Geometry: final body of the model. Coordinates: model frame, mm. Face numbers are marked on the shaded views. A direction names the side the tool comes from. Round coordinates to 2 decimals unless told otherwise and drop trailing zeros. Write each loop counter-clockwise with the first axis right and the second up, starting at its lowest first coordinate (ties: lowest second). Pieces come first, ordered by that corner, then holes. Notation, with made-up numbers: (78.5, -0.5) - (88.5, -0.5) arc R22 ccw to (88.5, 27.5) - close; hole circle Ø3 at (10, 12.25). An arc over 180 degrees is marked (long way). Use a Markdown table: item, result. Add a question column.
```python
from build123d import *

# Parameters (mm, degrees)
F0_R     = 28.575
F0_R_2   = 17.4625
F1_DEPTH = 61.976
F3_R     = 21.844
F4_DEPTH = 50.8
F7_R     = 1.5875
F8_DEPTH = 12.7


with BuildPart() as f1:
    # F0 (on Right) → F1 (new body)
    with BuildSketch(Plane.YZ):
        Circle(F0_R)
        Circle(F0_R_2, mode=Mode.SUBTRACT)
    extrude(amount=-F1_DEPTH)

    # F3 (on offset) → F4 (cut)
    with BuildSketch(Plane.YZ.offset(-5.588)):
        Circle(F3_R)
    extrude(amount=-F4_DEPTH, mode=Mode.SUBTRACT)

    # F7 (on face) → F8 (cut)
    with BuildSketch(Plane.XY.offset(28.575)):
        with Locations((-13.462, 0)):
            Circle(F7_R)
    extrude(amount=-F8_DEPTH, mode=Mode.SUBTRACT)


solid = f1.part
```
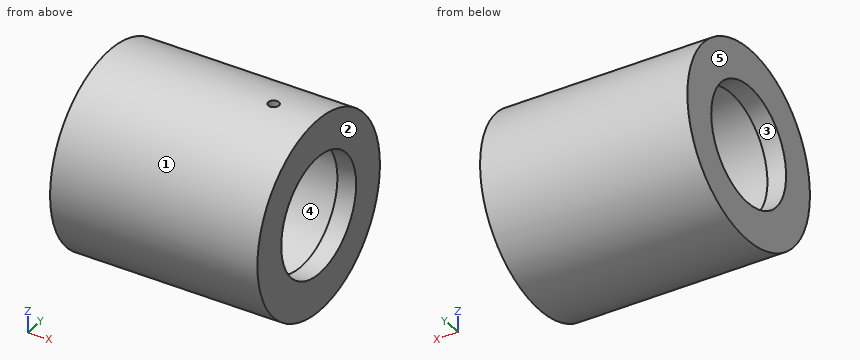
1) Section C-C, the plane y = -12. Return the cut outline in (x, z), then the cut area to 3 significant figures.
2) Set-up query: the marked faces 4 and 5. Return all of +Z, -Z, +X, -X, +Y, -Y with unobstructed straight access to the full face (end or side cutting, diameter ignored); none if empty.
3) Section B-B, the plane y = 0. Return the cut outline in (x, z) (1 decimal).
4) Material intervals for L1, parallel to X at y = 19.5, z = 8; L2, parallel to Z at x = -3.05, y = 0 (1 decimal); L3, parallel to Y at x = -11.5, z = -11.5, sorted ascending. Write a range as from..to.
5) Draft query along Z for the marked faces 1, 2 and 3. Return one class per face: released by +Z, released by -Z, zero draft, split by the parting line, or undercut.
6) Section A-A, the plane z = 0. Return the cut outline in (x, y) (1 decimal), then the cut area to 3 significant figures.
7) Pin query (flat end, axial travel): P1, Ø10, axis at x = -14, y = 6.5, coming from the +Z side; P2, Ø4, axis at x = -25, y = 7, coming from the -Z side; P3, Ø1.9, axis at x = -13.462, y = 0, coming from the +Z side; P4, Ø22, axis at y = 5.5, z = -1, coming from the -X side. Return the tip coordinate at first contact, or that it passes through.
8) Section D-D, the plane z = 23. Return the cut outline in (x, y) (1 decimal), then the cut area to 3 significant figures.
Output values:
| question | item | result |
|---|---|---|
| 1 | outline | (-61.98, -25.93) - (0, -25.93) - (0, -12.69) - (-5.59, -12.69) - (-5.59, -18.25) - (-56.39, -18.25) - (-56.39, -12.69) - (-61.98, -12.69) - close; (-61.98, 12.69) - (-56.39, 12.69) - (-56.39, 18.25) - (-5.59, 18.25) - (-5.59, 12.69) - (0, 12.69) - (0, 25.93) - (-61.98, 25.93) - close |
| 1 | area | 1,080 mm^2 |
| 2 | face 4 | none |
| 2 | face 5 | +Z, -Z, -X, +Y, -Y |
| 3 | outline | (-62, -28.6) - (0, -28.6) - (0, -17.5) - (-5.6, -17.5) - (-5.6, -21.8) - (-56.4, -21.8) - (-56.4, -17.5) - (-62, -17.5) - close; (-62, 17.5) - (-56.4, 17.5) - (-56.4, 21.8) - (-15, 21.8) - (-15, 28.6) - (-62, 28.6) - close; (-11.9, 21.8) - (-5.6, 21.8) - (-5.6, 17.5) - (0, 17.5) - (0, 28.6) - (-11.9, 28.6) - close |
| 4 | L1 | x = -61.98..-56.39, -5.59..0 |
| 4 | L2 | z = -28.6..-17.5, 17.5..28.6 |
| 4 | L3 | y = -26.16..-18.57, 18.57..26.16 |
| 5 | face 1 | split by the parting line |
| 5 | face 2 | zero draft |
| 5 | face 3 | undercut |
| 6 | outline | (-62, -28.6) - (0, -28.6) - (0, -17.5) - (-5.6, -17.5) - (-5.6, -21.8) - (-56.4, -21.8) - (-56.4, -17.5) - (-62, -17.5) - close; (-62, 17.5) - (-56.4, 17.5) - (-56.4, 21.8) - (-5.6, 21.8) - (-5.6, 17.5) - (0, 17.5) - (0, 28.6) - (-62, 28.6) - close |
| 6 | area | 932 mm^2 |
| 7 | P1 | stops at z = 28.54 |
| 7 | P2 | stops at z = -28.13 |
| 7 | P3 | stops at z = -21.82 |
| 7 | P4 | passes through |
| 8 | outline | (-62, -17) - (0, -17) - (0, 17) - (-62, 17) - close; hole circle Ø3.2 at (-13.5, 0) |
| 8 | area | 2,090 mm^2 |
